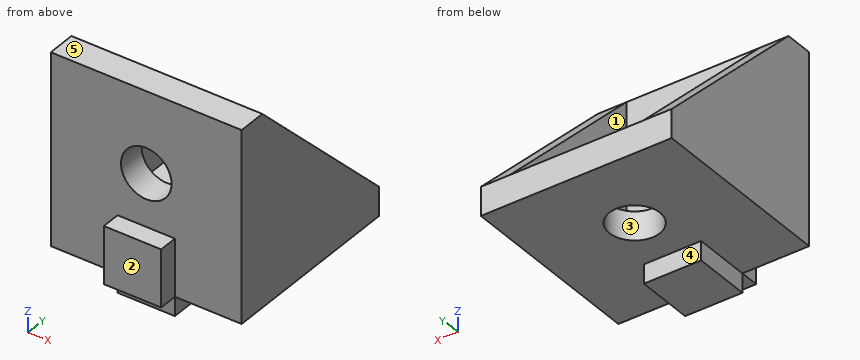
```python
from build123d import *

# Parameters (mm, degrees)
ESBO_O1_W                = 20
ESBO_O1_H                = 20
RESSALTO_EXTRUS_O1_DEPTH = 20
CORTE_EXTRUS_O1_DEPTH    = 21
ESBO_O3_W                = 14
ESBO_O3_H                = 17
CORTE_EXTRUS_O2_DEPTH    = 17
ESBO_O4_W                = 6
ESBO_O4_H                = 6
RESSALTO_EXTRUS_O2_DEPTH = 2
ESBO_O5_W                = 6
ESBO_O5_H                = 6
RESSALTO_EXTRUS_O3_DEPTH = 2
ESBO_O6_R                = 2.65
CORTE_EXTRUS_O3_DEPTH    = 6
ESBO_O7_R                = 2.65
CORTE_EXTRUS_O4_DEPTH    = 6


with BuildPart() as part:
    # Esboço1 → Ressalto-extrusão1 (new body)
    with BuildSketch(Plane.XY):
        with Locations((10, 10)):
            Rectangle(ESBO_O1_W, ESBO_O1_H)
    extrude(amount=RESSALTO_EXTRUS_O1_DEPTH)

    # Esboço2 → Corte-extrusão1 (cut, through all)
    with BuildSketch(Plane(origin=(20, 0, 0), x_dir=(0, 0, -1), z_dir=(1, 0, 0))):
        Polygon((-3, 20), (-20, 3), (-20, 20), align=None)
    extrude(amount=-CORTE_EXTRUS_O1_DEPTH, mode=Mode.SUBTRACT)

    # Esboço3 → Corte-extrusão2 (cut)
    with BuildSketch(Plane.XY.offset(20)):
        with Locations((10, 11.5)):
            Rectangle(ESBO_O3_W, ESBO_O3_H)
    extrude(amount=-CORTE_EXTRUS_O2_DEPTH, mode=Mode.SUBTRACT)

    # Esboço4 → Ressalto-extrusão2 (add)
    with BuildSketch(Plane(origin=(0, 0, 0), x_dir=(-1, 0, 0), z_dir=(0, 0, -1))):
        with Locations((-10, 3)):
            Rectangle(ESBO_O4_W, ESBO_O4_H)
    extrude(amount=RESSALTO_EXTRUS_O2_DEPTH)

    # Esboço5 → Ressalto-extrusão3 (add)
    with BuildSketch(Plane.XZ):
        with Locations((10, 3)):
            Rectangle(ESBO_O5_W, ESBO_O5_H)
    extrude(amount=RESSALTO_EXTRUS_O3_DEPTH)

    # Esboço6 → Corte-extrusão3 (cut, through all)
    with BuildSketch(Plane.XY.offset(3)):
        with Locations((10, 11.5)):
            Circle(ESBO_O6_R)
    extrude(amount=-CORTE_EXTRUS_O3_DEPTH, mode=Mode.SUBTRACT)

    # Esboço7 → Corte-extrusão4 (cut, through all)
    with BuildSketch(Plane(origin=(0, 3, 0), x_dir=(1, 0, 0), z_dir=(0, 1, 0))):
        with Locations((10, -11.5)):
            Circle(ESBO_O7_R)
    extrude(amount=-CORTE_EXTRUS_O4_DEPTH, mode=Mode.SUBTRACT)


solid = part.part
```
Check sheet for the modelled part. Datum: model origin and axes. Units: mm. Face numbers are marked on the shaded views. A direction names the side the tool comes from. Coordinates: 2 decimals unless noted, no trailing zeros. Write each loop counter-clockwise with the first axis right and the second up, starting at its lowest first coordinate (ties: lowest second). Pieces come first, ordered by that corner, then holes. Notation, with made-up numbers: M 84.25,70 L 126.25,70 A18 cw 126.25,89 Z; hole C 50.25,63 d5. An arc over 180 degrees is marked long. Write item = value, one per line. Start each with the question number.
1. Go/stop test with flat-tipped pins: pin 1 (0.6 mm diameter, centred on y = 2, z = -1, fed in from -X); pin 2 (8 mm diameter, centred on x = 18, z = 14, fed in from +Y); pin 3 (1.6 mm diameter, centred on x = 11, y = -1, fed in from -Z); pin 4 (3 mm diameter, centred on x = 10, z = 11.5, fed in from -Y). Record where each tip stops, or that it passes through.
2. Sectioned sample at C-C (x = 10). Record the cut outline in (y, z).
3. Sectioned sample at D-D (z = 17.5). Record the cut outline in (x, y), then the cut area to 3 significant figures.
4. Thickness scan on probe 1 along Z at (x, y) = (10, 1.3); probe 2 along X at (y, z) = (7.5, 4.75). Record the ranges inside material, lowest first.
5. Sectioned sample at A-A (z = 11.5). Record the cut outline in (x, y), then the cut area to 3 significant figures.
6. Tool access check on the marked faces 1 and 2. Record the directions out of +Z, -Z, +X, -X, +Y, -Y that give a thin tool (end or side, any length) a straight path to the whole face; none if there is none.
7. Mould release check, pull along Y, two halves, no side actions. Record for the marked faces 3, 4 and 5: pulls with the +Y half, pulls with the -Y half, needs draft (parallel to the pull), parting line crosses it, or undercut.
The answers:
q1.pin_1 = 7
q1.pin_2 = 13
q1.pin_3 = 0
q1.pin_4 = through
q2.outline = M -2,0 L 0,0 L 0,-2 L 6,-2 L 6,0 L 8.85,0 L 8.85,3 L 3,3 L 3,8.85 L 0,8.85 L 0,6 L -2,6 Z; M 0,14.15 L 3,14.15 L 3,20 L 0,20 Z; M 14.15,0 L 20,0 L 20,3 L 14.15,3 Z
q3.outline = M 0,0 L 20,0 L 20,5.5 L 17,5.5 L 17,3 L 3,3 L 3,5.5 L 0,5.5 Z
q3.area = 75.0 mm²
q4.probe_1 = -2 to 8.85, 14.15 to 20
q4.probe_2 = 0 to 3, 17 to 20
q5.outline = M 0,0 L 7.35,0 L 7.35,3 L 3,3 L 3,11.5 L 0,11.5 Z; M 12.65,0 L 20,0 L 20,11.5 L 17,11.5 L 17,3 L 12.65,3 Z
q5.area = 95.1 mm²
q6.face_1 = +Z, +Y
q6.face_2 = +Z, -Z, +X, -X, -Y
q7.face_3 = undercut
q7.face_4 = pulls with the +Y half
q7.face_5 = needs draft
